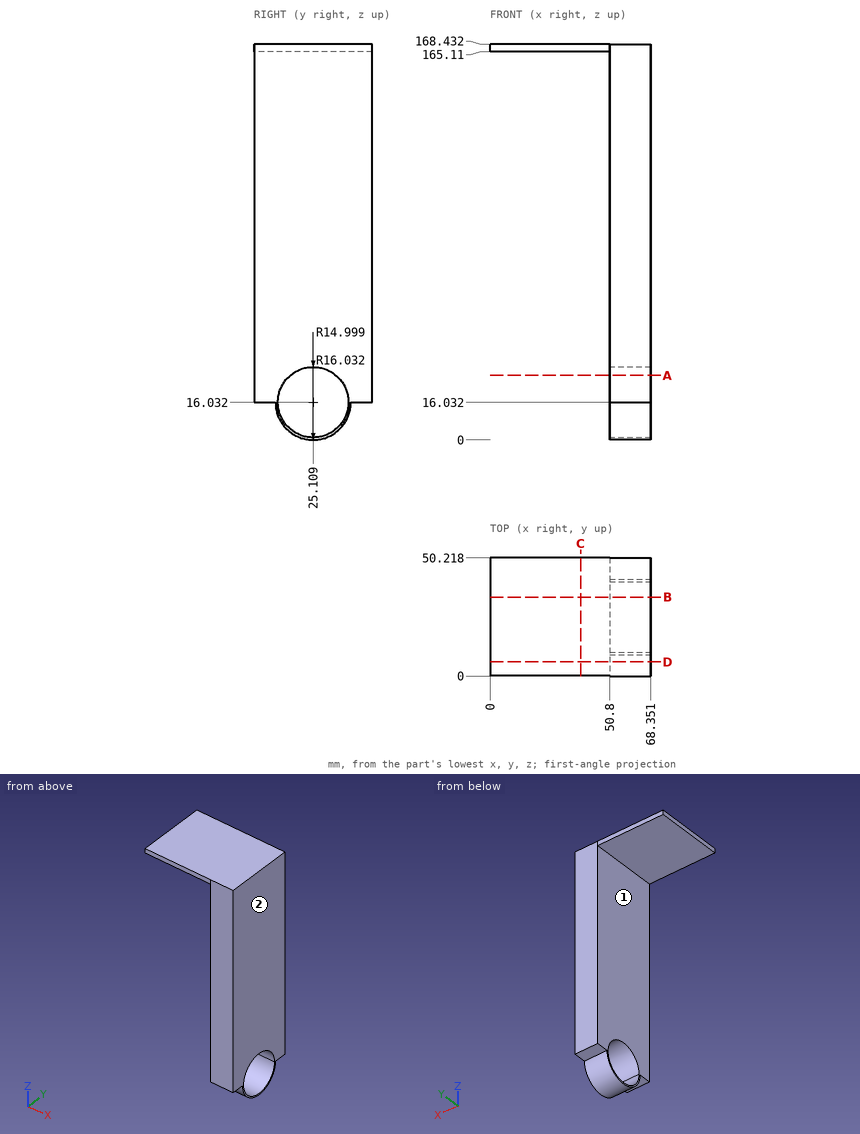
Source: three-view drawing plus pictorial views. Frame: mm from the lowest corner of the part. A direction names the side the tool comes from. Give positions to 0.01 mm unless a question says otherwise; leave off trailing zeros. Order: outer loops, then holes, each group sorted by start corner. A loop starts at its lowest first (then second) coordinate and runs counter-clockwise, first axis right, second up.
1. Material intervals for L1, parallel to X at y = 46.5, z = 120; L2, parallel to Z at x = 10, y = 37; L3, parallel to Z at x = 57.5, y = 7.5, sorted ascending.
Derived:
L1: x = 50.8 to 68.35
L2: z = 165.11 to 168.43
L3: z = 16.03 to 168.43
2. Section C-C on x = 38.5. Return the cut outline in (y, z).
Derived:
outline: (0, 165.11) - (50.22, 165.11) - (50.22, 168.43) - (0, 168.43) - close
3. Section A-A on z = 27.5. Return the cut outline in (x, y).
Derived:
outline: (50.8, 0) - (68.35, 0) - (68.35, 15.44) - (50.8, 15.44) - close; (50.8, 34.78) - (68.35, 34.78) - (68.35, 50.22) - (50.8, 50.22) - close
4. Section B-B on y = 33.5. Return the cut outline in (x, z) (1 decimal), and give its area (3 significant figures).
Derived:
outline: (0, 165.1) - (50.8, 165.1) - (50.8, 28.5) - (68.4, 28.5) - (68.4, 168.4) - (0, 168.4) - close; (50.8, 2.4) - (68.4, 2.4) - (68.4, 3.6) - (50.8, 3.6) - close
area: 2,650 mm2
5. Section D-D on y = 6. Return the cut outline in (x, z), and give its area (3 significant figures).
Derived:
outline: (0, 165.11) - (50.8, 165.11) - (50.8, 16.03) - (68.35, 16.03) - (68.35, 168.43) - (0, 168.43) - close
area: 2,840 mm2
6. Reachability of the marked faces 1 and 2 from +Z, -Z, +X, -X, +Y, -Y: full face, straight path, thin tool, end or side. Return the list, or none.
Derived:
face 1: -Z, -X, +Y, -Y
face 2: +Z, -Z, +X, +Y, -Y
7. Pin query (flat end, axial travel): pin 1 (15 mm diameter, centred on x = 19.5, y = 31.5, fed in from -Z); pin 2 (10 mm diameter, centred on x = 60.5, y = 4, fed in from -Z); pin 3 (1.5 mm diameter, centred on y = 7.5, z = 127, fed in from -X). Return the tip coordinate at first contact, or that it passes through.
Derived:
pin 1: stops at z = 165.11
pin 2: stops at z = 16.03
pin 3: stops at x = 50.8
